The listing builds one solid part. Answer for the finished solid, in the listing's coordinates (mm). A direction names the side the tool comes from. Round coordinates to 2 decimals unless told otherwise and drop trailing zeros. Order: outer loops, then holes, each group sorted by start corner. A loop starts at its lowest first (then second) coordinate and runs counter-clockwise, first axis right, second up. Notation, with made-up numbers: (-7, 13.25) -> (1, 13.25) arc R13 cw to (1, 34.25) -> close; hole circle Ø10 at (80, 70). An arc over 180 degrees is marked (long way). Return JSON: item names as keys, results as strings. Group by question number.
(1) Determine the mould class of faces 1 (the face through (45, -12, -20.5)), 2 (the face through (44, -12, 20.5)), 3 (the face through (54.5, -10, 28)), 4 (the face through (-1, -10, -35.5)) for opening direction Z: +Z half, -Z half, draft (parallel to the pull), parting line (faces both ways), or undercut.
(2) The part is cut by section C-C (z = -23). Determine the outline of the cut face in (x, y).
(3) The part is cut by section B-B (x = -44.5). Determine the outline of the cut face in (y, z), plus the area to 3 significant figures.
(4) Which of the six approach directions +Z, -Z, +X, -X, +Y, -Y give full straight-line access (tool end or side, diameter ignored) to faces 5 (the face through (34.5, -10, 0)), 6 (the face through (12.5, -17, 0)), 7 (the face through (-45, -5, 20.5)), 8 (the face through (-8, -6, 25)), 9 (the face through (41.2, -8.6, 27.9))?
(5) Each of these flat-tipped pins is pushed along its axis until it touches: pin 1 (12.5 mm diameter, centred on x = -3, z = -13, fed in from -Y); pin 2 (12 mm diameter, centred on y = -8.5, z = -13, fed in from +X); pin 3 (6 mm diameter, centred on y = -14, z = 15.5, fed in from -X); pin 4 (5 mm diameter, centred on x = -46, y = -9.5, fed in from +Z). Where does it stop, or does it pass through?
(6) The part is cut by section D-D (y = -3.5). Determine the outline of the cut face in (x, z).
(7) The part is cut by section A-A (y = -8.5). Count the separate pieces of the cut face and the enclosed holes in it, plus the area to 3 significant figures.
(8) Consider line 1 (Z direction, x = -6.5, y = -6.75); line 2 (X direction, y = -8.5, z = 32.25); line 3 (Z direction, x = -45, y = -1). Determine where each line is inside the solid, lowest interval first. Write a range as [from, to].
from build123d import *

# Parameters (mm, degrees)
F1_DEPTH = 20
F3_DEPTH = 7
F4_DEPTH = 3
F6_D     = 6.6
F6_DEPTH = 15.001
F8_D     = 6.6
F9_D     = 5


with BuildPart() as f1:
    # F0 (on Front) → F1 (new body)
    with BuildSketch(Plane.XZ):
        Polygon((54.5, 35.5), (-54.5, 35.5), (-54.5, 20.5), (-34.5, 20.5), (-34.5, 0), (-34.5, -20.5), (-54.5, -20.5), (-54.5, -35.5), (54.5, -35.5), (54.5, -20.5), (34.5, -20.5), (34.5, 0), (34.5, 20.5), (54.5, 20.5), align=None)
    extrude(amount=F1_DEPTH)

    # F2 (on face) → F3 (cut)
    with BuildSketch(Plane.XZ.offset(20)):
        Polygon((0, 30), (-12.5, 30), (-12.5, 0), (-12.5, -30), (0, -30), (12.5, -30), (12.5, 0), (12.5, 30), align=None)
    extrude(amount=-F3_DEPTH, mode=Mode.SUBTRACT)

    # F2 (on face) → F4 (cut)
    with BuildSketch(Plane.XZ.offset(20)):
        Polygon((-12.5, 0), (-12.5, 30), (-54.5, 30), (-54.5, 20.5), (-34.5, 20.5), (-34.5, -20.5), (-54.5, -20.5), (-54.5, -30), (-12.5, -30), align=None)
    extrude(amount=-F4_DEPTH, mode=Mode.SUBTRACT)

    # F6 (through all, one way)
    with BuildSketch(Plane(origin=(0, 0, 20.5), x_dir=(1, 0, 0), z_dir=(0, 0, -1))):
        with Locations((-44.5, 8.5), (44.5, 8.5)):
            Circle(F6_D / 2)
    extrude(amount=-F6_DEPTH, mode=Mode.SUBTRACT)

    # F8 (through all)
    with Locations(Plane.XY.offset(-20.5)):
        with Locations((-44.5, -8.5), (44.5, -8.5)):
            Hole(F8_D / 2)

    # F9 (through all)
    with Locations(Plane.XZ.offset(20)):
        with Locations((-6.5, 23), (-6.5, -23), (6.5, -23), (6.5, 23)):
            Hole(F9_D / 2)


solid = f1.part
Answer below:
{
 "1": {"face 1": "undercut", "face 2": "undercut", "face 3": "draft", "face 4": "-Z half"},
 "2": {"outline": "(-54.5, -17) -> (-12.5, -17) -> (-12.5, -13) -> (-9, -13) -> (-9, 0) -> (-54.5, 0) -> close; (-4, -13) -> (4, -13) -> (4, 0) -> (-4, 0) -> close; (9, -13) -> (12.5, -13) -> (12.5, -20) -> (54.5, -20) -> (54.5, 0) -> (9, 0) -> close; hole circle Ø6.6 at (-44.5, -8.5); hole circle Ø6.6 at (44.5, -8.5)"},
 "3": {"outline": "(-20, -35.5) -> (-11.8, -35.5) -> (-11.8, -20.5) -> (-17, -20.5) -> (-17, -30) -> (-20, -30) -> close; (-20, 30) -> (-17, 30) -> (-17, 20.5) -> (-11.8, 20.5) -> (-11.8, 35.5) -> (-20, 35.5) -> close; (-5.2, -35.5) -> (0, -35.5) -> (0, -20.5) -> (-5.2, -20.5) -> close; (-5.2, 20.5) -> (0, 20.5) -> (0, 35.5) -> (-5.2, 35.5) -> close", "area": "345 mm²"},
 "4": {"face 5": "+X, +Y, -Y", "face 6": "-Y", "face 7": "-X, +Y, -Y", "face 8": "+Y, -Y", "face 9": "+Z, -Z"},
 "5": {"pin 1": "stops at y = -13", "pin 2": "stops at x = 34.5", "pin 3": "stops at x = -34.5", "pin 4": "stops at z = 35.5"},
 "6": {"outline": "(-54.5, -35.5) -> (54.5, -35.5) -> (54.5, -20.5) -> (34.5, -20.5) -> (34.5, 20.5) -> (54.5, 20.5) -> (54.5, 35.5) -> (-54.5, 35.5) -> (-54.5, 20.5) -> (-34.5, 20.5) -> (-34.5, -20.5) -> (-54.5, -20.5) -> close; hole circle Ø5 at (-6.5, -23); hole circle Ø5 at (-6.5, 23); hole circle Ø5 at (6.5, -23); hole circle Ø5 at (6.5, 23)"},
 "7": {"separate pieces": "5", "enclosed holes": "4", "area": "5,620 mm²"},
 "8": {"line 1": "z = [-35.5, -25.5], [-20.5, 20.5], [25.5, 35.5]", "line 2": "x = [-54.5, -47.8], [-41.2, 41.2], [47.8, 54.5]", "line 3": "z = [-35.5, -20.5], [20.5, 35.5]"}
}
